Source: three-view drawing plus pictorial views. Frame: mm from the lowest corner of the part. Coordinates: 2 decimals unless noted, no trailing zeros. Write each loop counter-clockwise with the first axis right and the second up, starting at its lowest first coordinate (ties: lowest second). Pieces come first, ordered by that corner, then holes. Notation, with made-up numbers: M 14.25,30.25 L 66.25,30.25 A27 cw 66.25,61.25 Z; hole C 19.25,53.25 d3. An arc over 180 degrees is marked long. Use CSV: the item, a comma, the result in double quotes.
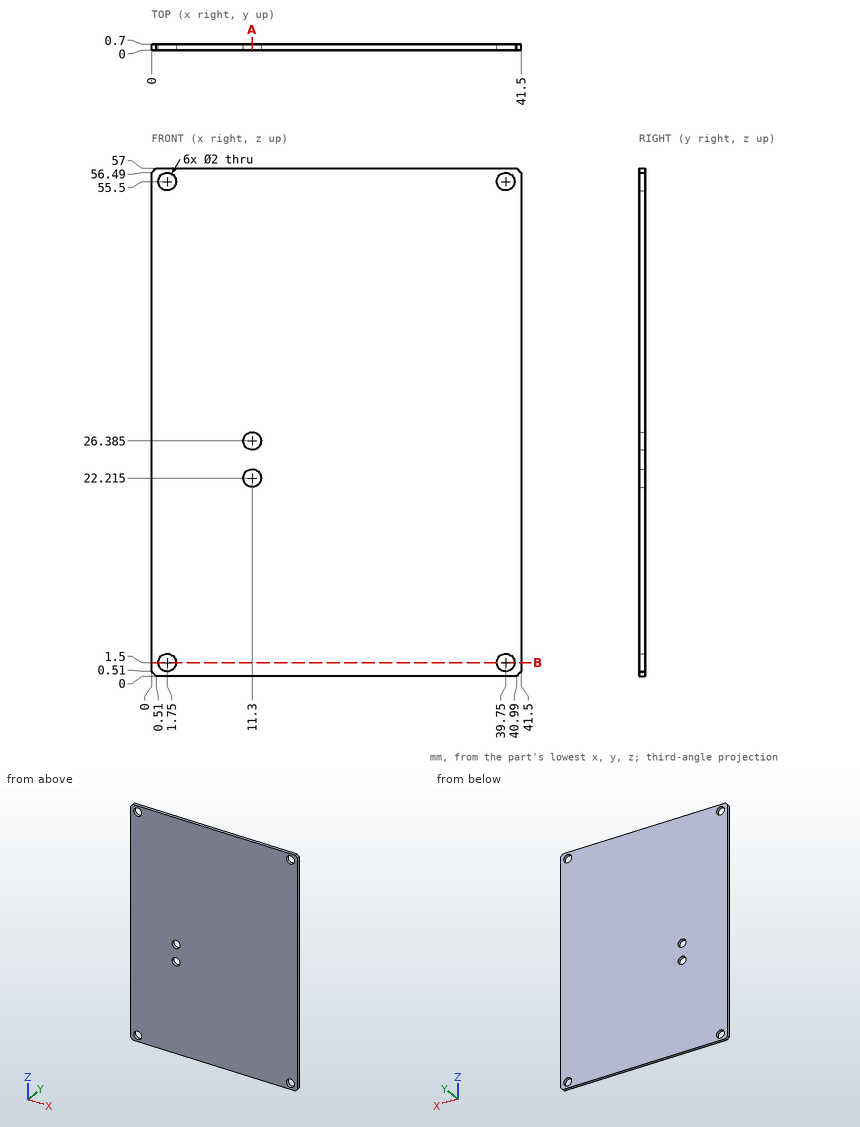
1. Section A-A (x = 11.3). Return loops of the section in (y, z) (1 decimal).
Resolved:
outline,"M 0,0 L 0.7,0 L 0.7,21.2 L 0,21.2 Z; M 0,23.2 L 0.7,23.2 L 0.7,25.4 L 0,25.4 Z; M 0,27.4 L 0.7,27.4 L 0.7,57 L 0,57 Z"
2. Section B-B (z = 1.5). Return loops of the section in (x, y).
Resolved:
outline,"M 0,0 L 0.75,0 L 0.75,0.7 L 0,0.7 Z; M 2.75,0 L 38.75,0 L 38.75,0.7 L 2.75,0.7 Z; M 40.75,0 L 41.5,0 L 41.5,0.7 L 40.75,0.7 Z"
3. Material intervals for line 1 (X direction, y = 0.2, z = 55.5); line 2 (Z direction, x = 11.3, y = 0.25) (1 decimal); line 3 (Z direction, x = 1.75, y = 0.5), sorted ascending. Write a range as [from, to].
Resolved:
line 1,"x = [0, 0.75], [2.75, 38.75], [40.75, 41.5]"
line 2,"z = [0, 21.2], [23.2, 25.4], [27.4, 57]"
line 3,"z = [0, 0.5], [2.5, 54.5], [56.5, 57]"
